Could you check a few things on this model? Use its own coordinates, in mm. A direction names the side the tool comes from. Coordinates: 2 decimals unless noted, no trailing zeros. Order: outer loops, then holes, each group sorted by start corner. A loop starts at its lowest first (then second) coordinate and runs counter-clockwise, first axis right, second up. Notation, with made-up numbers: M 39.5,10 L 92.5,10 A13 ccw 92.5,20 Z; hole C 44,32 d7. An arc over 180 degrees is marked long. Write item = value, one per line. Start each with the question number.
from build123d import *

# Parameters (mm, degrees)
BOSS_EXTRU_1_DEPTH      = 6
ESQUISSE2_R             = 20
ESQUISSE2_R_2           = 15
ENL_V_MAT_EXTRU_1_DEPTH = 3
ESQUISSE3_W             = 9.17
ESQUISSE3_H             = 20
BOSS_EXTRU_2_DEPTH      = 6
ESQUISSE4_R             = 1.5
ENL_V_MAT_EXTRU_2_DEPTH = 10


with BuildPart() as part:
    # Esquisse1 → Boss.-Extru.1 (new body)
    with BuildSketch(Plane.XY):
        with BuildLine():
            Line((42.613906887, 3.786407767), (42.613906887, 23.786407767))
            Line((42.613906887, 23.786407767), (-43.211335831, 23.786407767))
            ThreePointArc((-43.211335831, 23.786407767), (-29.069200208, 17.928543391), (-23.211335831, 3.786407767))
            Line((-23.211335831, 3.786407767), (42.613906887, 3.786407767))
        make_face()
        with BuildLine():
            ThreePointArc((-23.211335831, 3.786407767), (-29.069200208, 17.928543391), (-43.211335831, 23.786407767))
            Line((-43.211335831, 23.786407767), (-43.211335831, 18.786407767))
            ThreePointArc((-43.211335831, 18.786407767), (-32.604734113, 14.393009485), (-28.211335831, 3.786407767))
            Line((-28.211335831, 3.786407767), (-23.211335831, 3.786407767))
        make_face()
        with BuildLine():
            Line((-43.211335831, 18.786407767), (-43.211335831, 23.786407767))
            ThreePointArc((-43.211335831, 23.786407767), (-57.353471455, -10.355727857), (-23.211335831, 3.786407767))
            Line((-23.211335831, 3.786407767), (-28.211335831, 3.786407767))
            ThreePointArc((-28.211335831, 3.786407767), (-53.817937549, -6.820193951), (-43.211335831, 18.786407767))
        make_face()
    extrude(amount=BOSS_EXTRU_1_DEPTH)

    # Esquisse2 → Enlèv. mat.-Extru.1 (cut)
    with BuildSketch(Plane.XY.offset(6)):
        with Locations((-43.211335831, 3.786407767)):
            Circle(ESQUISSE2_R)
        with Locations((-43.211335831, 3.786407767)):
            Circle(ESQUISSE2_R_2, mode=Mode.SUBTRACT)
    extrude(amount=-ENL_V_MAT_EXTRU_1_DEPTH, mode=Mode.SUBTRACT)

    # Esquisse3 → Boss.-Extru.2 (add)
    with BuildSketch(Plane.XY.offset(6)):
        with Locations((47.198906887, 13.786407767)):
            Rectangle(ESQUISSE3_W, ESQUISSE3_H)
    extrude(amount=-BOSS_EXTRU_2_DEPTH)

    # Esquisse4 → Enlèv. mat.-Extru.2 (cut)
    with BuildSketch(Plane(origin=(0, 0, 0), x_dir=(-1, 0, 0), z_dir=(0, 0, -1))):
        with Locations((-48.783906887, 20.786407767)):
            Circle(ESQUISSE4_R)
        with Locations((-48.783906887, 6.786407767)):
            Circle(ESQUISSE4_R)
    extrude(amount=-ENL_V_MAT_EXTRU_2_DEPTH, mode=Mode.SUBTRACT)


solid = part.part
(1) Will these pins go through, and if not, where does the flat tip stop? P1, Ø3, axis at x = 18.5, z = 2, coming from the -Y side; P2, Ø2, axis at y = 13.5, z = 4.5, coming from the -X side; P3, Ø1.5, axis at y = -11, z = 1, coming from the +X side.
(2) Thinking about a two-plate mould opening in X: for faces 1 (the flat face through (-40, 19, 3)), 2 (the flat face through (51.784, 14, 3)), 3 (the cylindrical face through (47.353, 7.237, 2.958)), which applies, released by +X, released by -X, zero draft, split by the parting line, or undercut?
(3) Please list where these lines run through material, in increasing order: probe 1 along Y at (x, z) = (13, 5.4); probe 2 along X at (y, z) = (-8, 1.5); probe 3 along Z at (x, y) = (-51.5, -9). Write a range as from..to.
(4) Imagine slicing it at D-D on y = 1.5. List the corners of the cut face in (x, z) for me.
(5) Imagine slicing it at B-B on x = -44.5. List the corners of the cut face in (y, z) for me.
(6) Imagine slicing it at A-A on y = 15.5. List the corners of the cut face in (x, z) for me.
(7) Imagine slicing it at C-C on z = 1.3. List the corners of the cut face in (x, y) for me, plus the area to 3 significant figures.
(8) For faces 4 (the cylindrical face through (-28.91, 17.77, 4.52)), 5 (the flat face through (14, 3.786, 3)), 6 (the flat face through (4, 23.786, 3)), which set-ups out of +Z, -Z, +X, -X, +Y, -Y let a thin tool reach every point of the face, with its end or its side?
Response:
q1.P1 = 3.79
q1.P2 = -26.32
q1.P3 = -28.96
q2.face_1 = zero draft
q2.face_2 = released by +X
q2.face_3 = undercut
q3.probe_1 = 3.79..23.79
q3.probe_2 = -59.37..-52.49, -33.93..-27.05
q3.probe_3 = 0..3
q4.outline = M -63.08,0 L -58.04,0 L -58.04,3 L -63.08,3 Z; M -28.39,0 L -23.34,0 L -23.34,3 L -28.39,3 Z
q5.outline = M -16.17,0 L -11.16,0 L -11.16,3 L -16.17,3 Z; M 18.73,0 L 23.74,0 L 23.74,3 L 18.73,3 Z
q6.outline = M -59.42,0 L -52.58,0 L -52.58,3 L -59.42,3 Z; M -33.84,0 L 51.78,0 L 51.78,6 L -27,6 L -27,3 L -33.84,3 Z
q7.outline = M -43.21,23.79 A20 ccw long -23.21,3.79 L 51.78,3.79 L 51.78,23.79 Z; hole C -43.21,3.79 d30; hole C 48.78,6.79 d3; hole C 48.78,20.79 d3
q7.area = 2,120 mm2
q8.face_4 = +Z, -X, -Y
q8.face_5 = +Z, -Z, +X, -Y
q8.face_6 = +Z, -Z, +X, -X, +Y
